Could you check a few things on this drawing? It's one solid part, dimensions in mm from its lowest x, y, z. A direction names the side the tool comes from. Coordinates: 2 decimals unless noted, no trailing zeros. Order: outer loops, then holes, each group sorted by start corner. A loop starts at its lowest first (then second) coordinate and runs counter-clockwise, first axis right, second up. Notation, with made-up numbers: M -11,44 L -7,44 A13 cw -7,63 Z; hole C 74,85 d5. An arc over 180 degrees is marked long. Answer as CSV lines item,"result". Start each with the question number.
1. Will these pins go through, and if not, where does the flat tip stop? pin 1 (3 mm diameter, centred on x = 31.5, z = 40.5, fed in from -Y); pin 2 (1.6 mm diameter, centred on y = 1, z = 43.5, fed in from -X).
2. If we section it at A-A (z = 50): List the corners of the cut face in (x, y) for me, plus the area to 3 significant figures.
3. If we section it at B-B (x = 29): List the corners of the cut face in (y, z) for me.
4. If we section it at D-D (y = 16.25): List the corners of the cut face in (x, z) for me.
5. If we section it at C-C (y = 11): List the corners of the cut face in (x, z) for me, plus the area to 3 significant figures.
6. On a 3-axis mill with a long thin cutter (end or side, diameter ignored), from which of +Z, -Z, +X, -X, +Y, -Y can I reach the whole of each face in a straight line? I mean the marked faces 1, 2 and 3. Say none if no direction works.
7. I need wall thicknesses on line 1 along Z through (x, y) = (29, 11.5); line 2 along X through (y, z) = (17.75, 50); line 3 along X through (y, z) = (11, 8). Which ranges of each line are inside material? Lowest first, please. Write a range as from..to.
8. If we mould it in two halves opening along X, with no side actions, what happens to the marked faces 4, 5, 6 and 7? For each: released by +X, released by -X, zero draft, split by the parting line, or undercut.
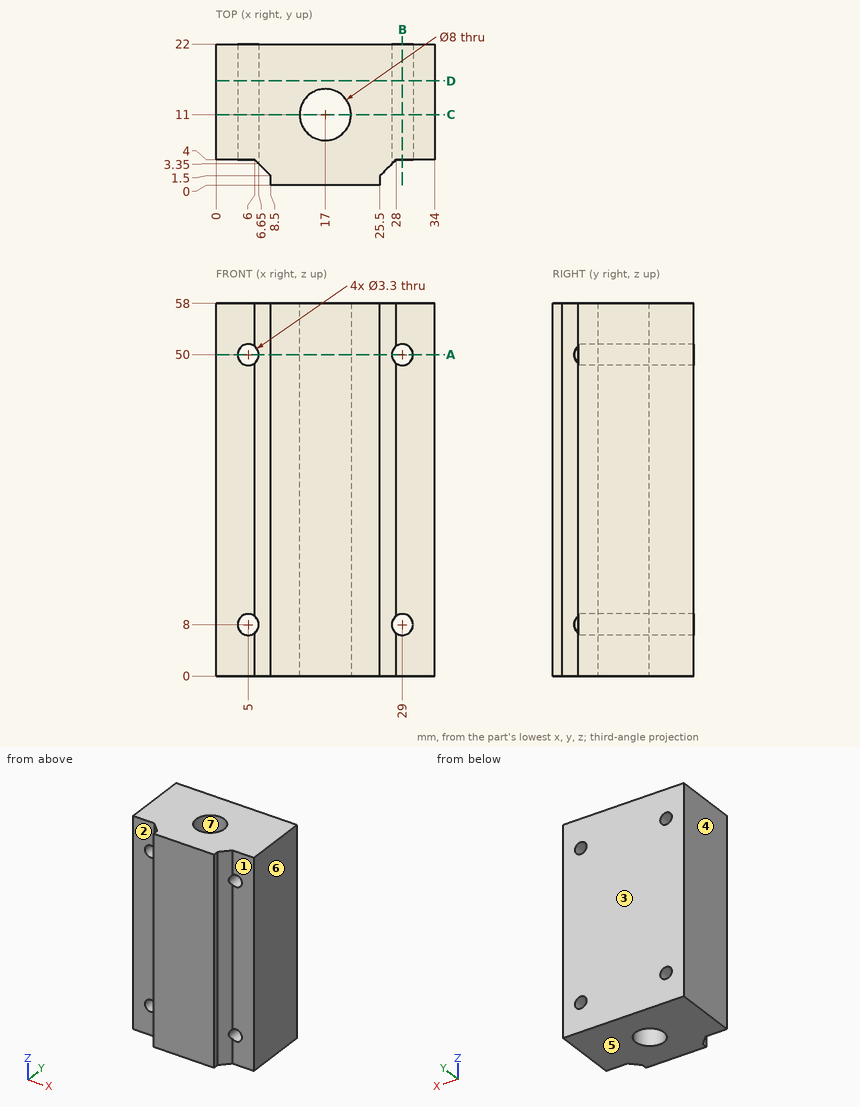
Solved:
1,pin 1,"y = 4"
1,pin 2,"x = 8.2"
2,outline,"M 0,4 L 3.35,4 L 3.35,22 L 0,22 Z; M 6.65,3.35 L 8.5,1.5 L 8.5,0 L 25.5,0 L 25.5,1.5 L 27.35,3.35 L 27.35,22 L 6.65,22 Z; M 30.65,4 L 34,4 L 34,22 L 30.65,22 Z; hole C 17,11 d8"
2,area,"517 mm²"
3,outline,"M 4,0 L 22,0 L 22,6.35 L 4,6.35 Z; M 4,9.65 L 22,9.65 L 22,48.35 L 4,48.35 Z; M 4,51.65 L 22,51.65 L 22,58 L 4,58 Z"
4,outline,"M 0,0 L 34,0 L 34,58 L 0,58 Z; hole C 5,8 d3.3; hole C 5,50 d3.3; hole C 29,8 d3.3; hole C 29,50 d3.3"
5,outline,"M 0,0 L 13,0 L 13,58 L 0,58 Z; M 21,0 L 34,0 L 34,58 L 21,58 Z; hole C 5,8 d3.3; hole C 5,50 d3.3; hole C 29,8 d3.3; hole C 29,50 d3.3"
5,area,"1,470 mm²"
6,face 1,"+Z, -Z, +X, -Y"
6,face 2,"+Z, -Z, -X, -Y"
6,face 3,"+Z, -Z, +X, -X, +Y"
7,line 1,"0..6.35, 9.65..48.35, 51.65..58"
7,line 2,"0..3.35, 6.65..27.35, 30.65..34"
7,line 3,"0..3.35, 6.65..13, 21..27.35, 30.65..34"
8,face 4,"released by -X"
8,face 5,"zero draft"
8,face 6,"released by +X"
8,face 7,"undercut"
